```python
from build123d import *

# Parameters (mm, degrees)
CYLINDER002_R     = 2
CYLINDER002_DEPTH = 10
BOX002_W          = 5
BOX002_H          = 10
BOX002_DEPTH      = 18
EXTRUDE_DEPTH     = 10


with BuildPart() as cylinder002:
    # Cylinder002 → Cylinder002 (new body)
    with BuildSketch(Plane(origin=(-65, -38, 3.5), x_dir=(0, 0, -1), z_dir=(1, 0, 0))):
        Circle(CYLINDER002_R)
    extrude(amount=CYLINDER002_DEPTH)


with BuildPart() as cut002:
    # Box002 → Box002 (new body)
    with BuildSketch(Plane(origin=(-63, -43, -11), x_dir=(1, 0, 0), z_dir=(0, 0, 1))):
        with Locations((2.5, 5)):
            Rectangle(BOX002_W, BOX002_H)
    extrude(amount=BOX002_DEPTH)

    # Cut002: cut Cylinder002
    add(cylinder002.part, mode=Mode.SUBTRACT)


with BuildPart() as fusion001:
    # Sketch → Extrude (new body)
    with BuildSketch(Plane.XZ):
        Polygon((-49.224583, -10.083495), (-33.224583, -10.083495), (-33.224583, -6.313495), (-35.224583, -6.313495), (-49.224583, -7.313495), align=None)
    extrude(amount=EXTRUDE_DEPTH)


with BuildPart() as fusion001_1:
    # Extrude placement: moved
    add(fusion001.part.moved(Location((-8.775417, -33, -0.916505))))

    # Fusion001: union Cut002
    add(cut002.part)


solid = fusion001_1.part
```
Part model, mm, in its own coordinate system. A direction names the side the tool comes from. Give positions to 0.01 mm unless a question says otherwise; leave off trailing zeros. Write each loop counter-clockwise with the first axis right and the second up, starting at its lowest first coordinate (ties: lowest second). Pieces come first, ordered by that corner, then holes. Notation, with made-up numbers: (-39.75, -9) -> (7.25, -9) arc R16 ccw to (7.25, 2) -> close; hole circle Ø7 at (85, -28). An arc over 180 degrees is marked (long way). Put each result on its own line as item: value. Start each with the question number.
Item 1: Cut at C-C (x = -58.5). List the corners of the cut face in (y, z), then the cut area to 3 significant figures.
Item 2: Cut at D-D (y = -38). List the corners of the cut face in (x, z).
Item 3: Pin check, flat tips, straight feed: pin 1 Ø3 at (x, y) = (-46, -35) entering from +Z; pin 2 Ø1 at (x, y) = (-43, -39) entering from +Z; pin 3 Ø3 at (y, z) = (-39.5, -4.5) entering from +X. Stop position of each tip, or through.
Item 4: Cut at A-A (z = 3.5). List the corners of the cut face in (x, y), then the cut area to 3 significant figures.
Item 5: Cut at B-B (y = -41.5). List the corners of the cut face in (x, z), then the cut area to 3 significant figures.
Item 6: Which spindle directions (+Z, -Z, +X, -X, +Y, -Y) get a long thin tool onto all of the face, cutting with end or side? Do faces 4 (the face through (-43, -38, -7.23)), 5 (the face through (-61, -38, 7)). Say none if no direction does.
Item 7: Pull direction Z, two halves, no side cores. Call faces 1 (the face through (-60.535, -39.952, 3.934)), 2 (the face through (-50.902, -37.93, -7.723)), 3 (the face through (-58, -38, -1)): pulls with the +Z half, pulls with the -Z half, needs draft (parallel to the pull), parting line crosses it, or undercut.
Item 8: Wall check: L1, parallel to Z at x = -60.95, y = -38; L2, parallel to Y at x = -61.6, z = 3.5; L3, parallel to X at y = -38.75, z = 1.25. Give the ranges that are in metal, low to high. Write a range as [from, to].
Answer list:
1. outline: (-43, -11) -> (-33, -11) -> (-33, 7) -> (-43, 7) -> close; hole circle Ø4 at (-38, 3.5)
1. area: 167 mm2
2. outline: (-63, -11) -> (-42, -11) -> (-42, -7.23) -> (-44, -7.23) -> (-58, -8.23) -> (-58, 1.5) -> (-63, 1.5) -> close; (-63, 5.5) -> (-58, 5.5) -> (-58, 7) -> (-63, 7) -> close
3. pin 1: stops at z = -7.27
3. pin 2: stops at z = -7.23
3. pin 3: stops at x = -58
4. outline: (-63, -43) -> (-58, -43) -> (-58, -40) -> (-63, -40) -> close; (-63, -36) -> (-58, -36) -> (-58, -33) -> (-63, -33) -> close
4. area: 30.0 mm2
5. outline: (-63, -11) -> (-42, -11) -> (-42, -7.23) -> (-44, -7.23) -> (-58, -8.23) -> (-58, 7) -> (-63, 7) -> close
5. area: 143 mm2
6. face 4: +Z, +X, +Y, -Y
6. face 5: +Z, +X, -X, +Y, -Y
7. face 1: undercut
7. face 2: pulls with the +Z half
7. face 3: needs draft
8. L1: z = [-11, 1.5], [5.5, 7]
8. L2: y = [-43, -40], [-36, -33]
8. L3: x = [-63, -58]
